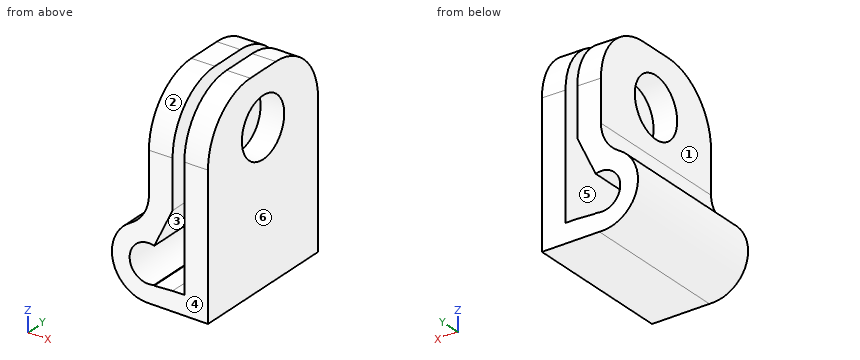
from build123d import *

# Parameters (mm, degrees)
F1_DEPTH = 13
F2_R     = 1.6
F3_DEPTH = 25
F5_DEPTH = 25
F6_R     = 3
F7_R     = 5
F8_R     = 2.5
F9_DEPTH = 25


with BuildPart() as f1:
    # F0 (on Front) → F1 (new body)
    with BuildSketch(Plane.XZ):
        with BuildLine():
            Line((-4.862412, 0.061252), (0, 0))
            Line((0, 0), (0, 17))
            Line((0, 17), (-2, 17))
            Line((-2, 17), (-2, 1.645369))
            Line((-2, 1.645369), (-3, 1.645369))
            Line((-3, 1.645369), (-3, 17))
            Line((-3, 17), (-5, 17))
            Line((-5, 17), (-5, 6.256132))
            ThreePointArc((-5, 6.256132), (-8.135924, 3.087515), (-4.862412, 0.061252))
        make_face()
    extrude(amount=F1_DEPTH)

    # F2 (on face) → F3 (cut)
    with BuildSketch(Plane.XZ.offset(13)):
        with Locations((-5.036688, 3.156349)):
            Circle(F2_R)
    extrude(amount=-F3_DEPTH, mode=Mode.SUBTRACT)

    # F4 (on face) → F5 (cut)
    with BuildSketch(Plane.XZ.offset(13)):
        Polygon((-2.599795, 8.748447), (-4.55274, 4.681404), (-4.59475, 3.031561), (-2.599795, 3.031561), align=None)
        Polygon((-2.599795, 3.031561), (-4.59475, 3.031561), (-4.55274, 1.576295), (-3, 1.645369), align=None)
    extrude(amount=-F5_DEPTH, mode=Mode.SUBTRACT)

    # F6
    f6_edges = [f1.edges().sort_by_distance(p)[0] for p in [
        (-5, -6.5, 6.256132),
    ]]
    fillet(f6_edges, radius=F6_R)

    # F7
    f7_edges = [f1.edges().sort_by_distance(p)[0] for p in [
        (-4, 0, 17),
        (-1, 0, 17),
        (-4, -13, 17),
        (-1, -13, 17),
    ]]
    fillet(f7_edges, radius=F7_R)

    # F8 (on face) → F9 (cut)
    with BuildSketch(Plane(origin=(-5, 0, 0), x_dir=(0, -1, 0), z_dir=(-1, 0, 0))):
        with Locations((6.5, 12.515542)):
            Circle(F8_R)
    extrude(amount=-F9_DEPTH, mode=Mode.SUBTRACT)


solid = f1.part
Model file for the job. Use its own axes, mm. Face numbers are marked on the shaded views. A direction names the side the tool comes from. Coordinates: 2 decimals unless noted, no trailing zeros. Write each loop counter-clockwise with the first axis right and the second up, starting at its lowest first coordinate (ties: lowest second). Pieces come first, ordered by that corner, then holes. Notation, with made-up numbers: (69.25, -10.75) -> (95.25, -10.75) arc R32 cw to (95.25, 18.25) -> close; hole circle Ø1 at (-26, 66). An arc over 180 degrees is marked (long way). One line per item, written item: value. Start each with the question number.
1) Flat gauge pins, fed straight in: pin 1 Ø6.5 at (y, z) = (-6.5, 12.52) entering from -X; pin 2 Ø0.5 at (x, y) = (-2.5, -4.5) entering from +Z; pin 3 Ø2.5 at (x, z) = (-5.04, 3.16) entering from +Y; pin 4 Ø1.5 at (x, z) = (-5, 15) entering from +Y. Where does each tip first touch, or does it go through?
2) Slice it at D-D on y = -1. Write the cut outline in (x, z).
3) Slice it at C-C on z = 8.25. Write the cut outline in (x, y), then the cut area to 3 significant figures.
4) Probe probe 1 along X at (y, z) = (-1.5, 13.75); probe 2 along Z at (x, y) = (-3.35, -6.5); probe 3 along Z at (x, y) = (-3.75, -6). List the from-to ranges inside material, lowest first.
5) Which spindle directions (+Z, -Z, +X, -X, +Y, -Y) get a long thin tool onto all of the face, cutting with end or side? Do the marked faces 1, 2 and 3. Say none if no direction does.
6) Slice it at A-A on y = -6.5. Write the cut outline in (x, z), then the cut area to 3 significant figures.
7) Slice it at B-B on z = 14.5. Write the cut outline in (x, y).
8) Pull direction X, two halves, no side cores. Call the marked faces 4, 5 and 6: +X half, -X half, draft (parallel to the pull), parting line (faces both ways), or undercut.
Answers follow:
1. pin 1: x = -5
1. pin 2: z = 1.65
1. pin 3: through
1. pin 4: y = -0.53
2. outline: (-6.54, 5.87) arc R3.1 ccw to (-4.86, 0.06) -> (0, 0) -> (0, 15) -> (-2, 15) -> (-2, 1.65) -> (-3, 1.65) -> (-4.55, 1.58) -> (-4.55, 1.63) arc R1.6 cw (long way) to (-4.55, 4.68) -> (-3, 7.92) -> (-3, 15) -> (-5, 15) -> (-5, 8.49) arc R3 cw to start
3. outline: (-5.01, -13) -> (-3, -13) -> (-3, 0) -> (-5.01, 0) -> close; (-2, -13) -> (0, -13) -> (0, 0) -> (-2, 0) -> close
3. area: 52.1 mm2
4. probe 1: -5 to -3, -2 to 0
4. probe 2: 0.04 to 1.63, 7.19 to 10.02, 15.02 to 17
4. probe 3: 0.05 to 1.61, 6.35 to 10.07, 14.97 to 17
5. face 1: +Z, -X, +Y, -Y
5. face 2: +Z, +X, -X, -Y
5. face 3: +Y, -Y
6. outline: (-6.54, 5.87) arc R3.1 ccw to (-4.86, 0.06) -> (0, 0) -> (0, 10.02) -> (-2, 10.02) -> (-2, 1.65) -> (-3, 1.65) -> (-4.55, 1.58) -> (-4.55, 1.63) arc R1.6 cw (long way) to (-4.55, 4.68) -> (-3, 7.92) -> (-3, 10.02) -> (-5, 10.02) -> (-5, 8.49) arc R3 cw to start; (-5, 15.02) -> (-3, 15.02) -> (-3, 17) -> (-5, 17) -> close; (-2, 15.02) -> (0, 15.02) -> (0, 17) -> (-2, 17) -> close
6. area: 52.7 mm2
7. outline: (-5, -12.33) -> (-3, -12.33) -> (-3, -8.02) -> (-5, -8.02) -> close; (-5, -4.98) -> (-3, -4.98) -> (-3, -0.67) -> (-5, -0.67) -> close; (-2, -12.33) -> (0, -12.33) -> (0, -8.02) -> (-2, -8.02) -> close; (-2, -4.98) -> (0, -4.98) -> (0, -0.67) -> (-2, -0.67) -> close
8. face 4: draft
8. face 5: undercut
8. face 6: +X half
